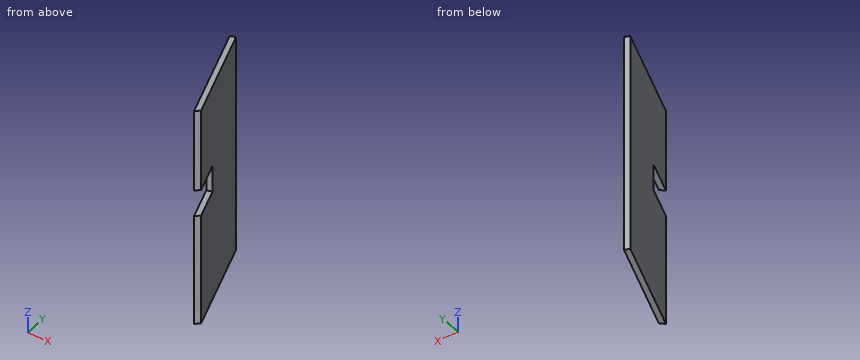
from build123d import *

# Parameters (mm, degrees)
BOSS_EXTRUDE1_DEPTH = 208.295833
SKETCH3_W           = 25
SKETCH3_H           = 33
CUT_EXTRUDE1_DEPTH  = 36.788128275


with BuildPart() as part:
    # Sketch2 → Boss-Extrude1 (new body)
    with BuildSketch(Plane.XY.offset(2)):
        Polygon((3386.129332678, -6568.675675181), (3418.890080551, -6658.762542636), (3422.744518293, -6654.731505307), (3390.828268184, -6566.966872936), align=None)
    extrude(amount=BOSS_EXTRUDE1_DEPTH)

    # Sketch3 → Cut-Extrude1 (cut, through all)
    with BuildSketch(Plane(origin=(885.586873602, 322.050140106, 0), x_dir=(0, 0, -1), z_dir=(0.939787101, 0.341760449, 0))):
        with Locations((-120, -7409.760556288)):
            Rectangle(SKETCH3_W, SKETCH3_H)
    extrude(amount=-CUT_EXTRUDE1_DEPTH, mode=Mode.SUBTRACT)


solid = part.part
Work out the finished part from the listing and answer in its coordinate system (mm). Coordinates: 2 decimals unless noted, no trailing zeros. Write each loop counter-clockwise with the first axis right and the second up, starting at its lowest first coordinate (ties: lowest second). Pieces come first, ordered by that corner, then holes. Notation, with made-up numbers: M 53.5,-34 L 112.5,-34 A16 ccw 112.5,-7 Z; hole C 23,-17.5 d6. An arc over 180 degrees is marked long. Write item = value, one per line.
1. The part is cut by section A-A (y = -6633.5). Determine the outline of the cut face in (x, z).
Solution:
outline = M 3409.7,2 L 3415.02,2 L 3415.02,107.5 L 3409.7,107.5 Z; M 3409.7,132.5 L 3415.02,132.5 L 3415.02,210.3 L 3409.7,210.3 Z
2. Flat-ended cylindrical pins translate along their axes: pin 1 (12 mm diameter, centred on y = -6636, z = 53.5, fed in from -X); pin 2 (1.5 mm diameter, centred on y = -6639.5, z = 147.5, fed in from -X); pin 3 (1.5 mm diameter, centred on y = -6595.5, z = 103.5, fed in from +X). Find the tip coordinate at first contact, or state that the pin passes through.
Solution:
pin_1 = 3408.43
pin_2 = 3411.61
pin_3 = 3401.48
3. The part is cut by section C-C (x = 3401). Determine the outline of the cut face in (y, z).
Solution:
outline = M -6609.57,2 L -6594.94,2 L -6594.94,210.3 L -6609.57,210.3 Z
4. The part is cut by section B-B (z = 181.5). Determine the outline of the cut face in (x, y).
Solution:
outline = M 3386.13,-6568.68 L 3418.89,-6658.76 L 3422.74,-6654.73 L 3390.83,-6566.97 Z
5. Straight lines are drawn through the part: line 1 (Z direction, x = 3412, y = -6633); line 2 (X direction, y = -6608.5, z = 132.5); line 3 (X direction, y = -6615, z = 170). For each, find the intervals that lie inside material, in ascending order. Write a range as from..to.
Solution:
line_1 = 2..107.5, 132.5..210.3
line_2 = 3400.61..3405.93
line_3 = 3402.98..3408.3
